Geometry check sheet. Reference: the model listing, model coordinates, mm. Face numbers are marked on the shaded views. Give positions to 0.01 mm unless a question says otherwise; leave off trailing zeros. Write each loop counter-clockwise with the first axis right and the second up, starting at its lowest first coordinate (ties: lowest second). Pieces come first, ordered by that corner, then holes. Notation, with made-up numbers: (29, 55) - (43, 55) arc R35 ccw to (43, 89) - close; hole circle Ø10 at (-2, 26.5). An arc over 180 degrees is marked (long way). Use a Markdown table: item, result.
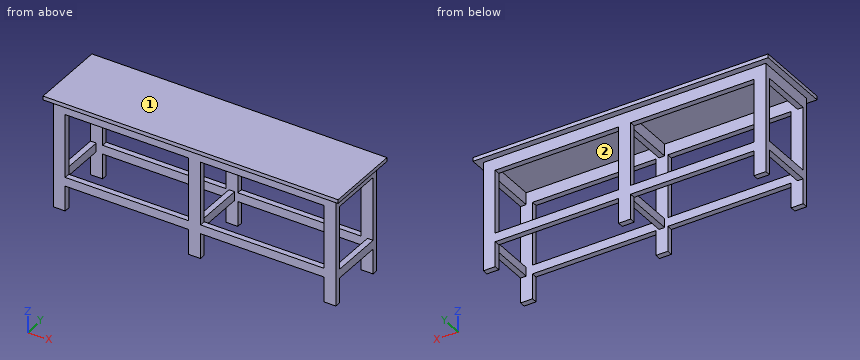
```python
from build123d import *

# Parameters (mm, degrees)
F1_W     = 2350
F1_H     = 610
F2_DEPTH = 30
F3_W     = 45
F3_H     = 420
F3_W_2   = 982.5
F3_H_2   = 45
F4_DEPTH = 95
F5_DEPTH = 870
F7_W     = 982.5
F7_H     = 45
F7_W_2   = 45
F7_H_2   = 420
F8_DEPTH = 70


# Not quite as in the source:
# - a feature names something its author has since deleted; it is built from what else it names


with BuildPart() as f2:
    # F1 (on offset) → F2 (new body)
    with BuildSketch(Plane.XY.offset(900)):
        Rectangle(F1_W, F1_H)
    extrude(amount=-F2_DEPTH)

    # F3 (on face) → F4 (join)
    with BuildSketch(Plane(origin=(0, 0, 870), x_dir=(1, 0, 0), z_dir=(0, 0, -1))):
        with Locations((-1102.5, 0)):
            Rectangle(F3_W, F3_H)
        with Locations((1102.5, 0)):
            Rectangle(F3_W, F3_H)
        with Locations((-538.75, 232.5)):
            Rectangle(F3_W_2, F3_H_2)
        with Locations((-538.75, -232.5)):
            Rectangle(F3_W_2, F3_H_2)
        Polygon((22.5, 210), (-22.5, 210), (-22.5, -210), (22.5, -210), (22.5, -47.5), (22.5, 47.5), align=None)
        with Locations((538.75, 232.5)):
            Rectangle(F3_W_2, F3_H_2)
        with Locations((538.75, -232.5)):
            Rectangle(F3_W_2, F3_H_2)
    extrude(amount=F4_DEPTH)

    # F3 (on face) → F5 (join)
    with BuildSketch(Plane(origin=(0, 0, 870), x_dir=(1, 0, 0), z_dir=(0, 0, -1))):
        Polygon((-1030, 255), (-1125, 255), (-1125, 210), (-1080, 210), (-1030, 210), align=None)
        Polygon((47.5, 255), (-47.5, 255), (-47.5, 210), (-22.5, 210), (22.5, 210), (47.5, 210), align=None)
        Polygon((-1080, -210), (-1125, -210), (-1125, -255), (-1030, -255), (-1030, -210), align=None)
        Polygon((1125, 255), (1030, 255), (1030, 210), (1080, 210), (1125, 210), align=None)
        Polygon((22.5, -210), (-22.5, -210), (-47.5, -210), (-47.5, -255), (47.5, -255), (47.5, -210), align=None)
        Polygon((1125, -210), (1080, -210), (1030, -210), (1030, -255), (1125, -255), align=None)
    extrude(amount=F5_DEPTH)

    # F7 (on offset) → F8 (join)
    with BuildSketch(Plane.XY.offset(200)):
        with Locations((-538.75, 232.5)):
            Rectangle(F7_W, F7_H)
        Polygon((22.5, 255), (-47.5, 255), (-47.5, 210), (-22.5, 210), (22.5, 210), (47.5, 210), (47.5, 255), align=None)
        Polygon((67.5, 255), (47.5, 255), (47.5, 210), (67.5, 210), (1030, 210), (1030, 255), align=None)
        Polygon((22.5, 210), (-22.5, 210), (-22.5, -210), (22.5, -210), (22.5, -47.5), (22.5, 47.5), align=None)
        Polygon((22.5, -210), (-22.5, -210), (-47.5, -210), (-47.5, -255), (22.5, -255), (47.5, -255), (47.5, -210), align=None)
        with Locations((-538.75, -232.5)):
            Rectangle(F7_W, F7_H)
        Polygon((67.5, -210), (47.5, -210), (47.5, -255), (1030, -255), (1030, -210), align=None)
        with Locations((-1102.5, 0)):
            Rectangle(F7_W_2, F7_H_2)
        with Locations((1102.5, 0)):
            Rectangle(F7_W_2, F7_H_2)
    extrude(amount=F8_DEPTH)


solid = f2.part
```
1) Section check B-B on z = 318. Record the boundary of the cut face in (x, y), then the cut area to 4 significant figures.
Working result:
| item | result |
|---|---|
| outline | (-1125, -255) - (-1030, -255) - (-1030, -210) - (-1125, -210) - close; (-1125, 210) - (-1030, 210) - (-1030, 255) - (-1125, 255) - close; (-47.5, -255) - (47.5, -255) - (47.5, -210) - (-47.5, -210) - close; (-47.5, 210) - (47.5, 210) - (47.5, 255) - (-47.5, 255) - close; (1030, -255) - (1125, -255) - (1125, -210) - (1030, -210) - close; (1030, 210) - (1125, 210) - (1125, 255) - (1030, 255) - close |
| area | 25,650 mm² |
2) Section check D-D on y = 232. Record the boundary of the cut face in (x, z).
Working result:
| item | result |
|---|---|
| outline | (-1175, 870) - (-1125, 870) - (-1125, 0) - (-1030, 0) - (-1030, 200) - (-47.5, 200) - (-47.5, 0) - (47.5, 0) - (47.5, 200) - (1030, 200) - (1030, 0) - (1125, 0) - (1125, 870) - (1175, 870) - (1175, 900) - (-1175, 900) - close; hole (-1030, 270) - (-47.5, 270) - (-47.5, 775) - (-1030, 775) - close; hole (47.5, 270) - (1030, 270) - (1030, 775) - (47.5, 775) - close |
3) Section check C-C on y = -19. Record the boundary of the cut face in (x, z), then the cut area to 3 significant figures.
Working result:
| item | result |
|---|---|
| outline | (-1175, 870) - (-1125, 870) - (-1125, 775) - (-1080, 775) - (-1080, 870) - (-22.5, 870) - (-22.5, 775) - (22.5, 775) - (22.5, 870) - (1080, 870) - (1080, 775) - (1125, 775) - (1125, 870) - (1175, 870) - (1175, 900) - (-1175, 900) - close; (-1125, 200) - (-1080, 200) - (-1080, 270) - (-1125, 270) - close; (-22.5, 200) - (22.5, 200) - (22.5, 270) - (-22.5, 270) - close; (1080, 200) - (1125, 200) - (1125, 270) - (1080, 270) - close |
| area | 92,800 mm² |
4) Section check A-A on x = 374. Record the boundary of the cut face in (y, z).
Working result:
| item | result |
|---|---|
| outline | (-305, 870) - (-255, 870) - (-255, 775) - (-210, 775) - (-210, 870) - (210, 870) - (210, 775) - (255, 775) - (255, 870) - (305, 870) - (305, 900) - (-305, 900) - close; (-255, 200) - (-210, 200) - (-210, 270) - (-255, 270) - close; (210, 200) - (255, 200) - (255, 270) - (210, 270) - close |
5) Material ranges on L1, parallel to X at y = -245.5, z = 721; L2, parallel to X at y = -129.5, z = 237.5; L3, parallel to Z at x = 970, y = -213.5, recorded low to high. Write a range as from..to.
Working result:
| item | result |
|---|---|
| L1 | x = -1125..-1030, -47.5..47.5, 1030..1125 |
| L2 | x = -1125..-1080, -22.5..22.5, 1080..1125 |
| L3 | z = 200..270, 775..900 |
6) Depth check by flat-ended pin: P1, Ø4, axis at x = 403.5, y = 115.5, coming from the -Z side; P2, Ø13.5, axis at x = 1092, y = -16, coming from the -Z side; P3, Ø22.5, axis at y = -233.5, z = 55, coming from the +X side. Enter the tip coordinate at first touch or a pass-through.
Working result:
| item | result |
|---|---|
| P1 | stops at z = 870 |
| P2 | stops at z = 200 |
| P3 | stops at x = 1125 |
7) Mould release check, pull along Y, two halves, no side actions. Record for the marked faces 1 and 2: pulls with the +Y half, pulls with the -Y half, needs draft (parallel to the pull), parting line crosses it, or undercut.
Working result:
| item | result |
|---|---|
| face 1 | needs draft |
| face 2 | undercut |
